```python
from build123d import *

# Parameters (mm, degrees)
BOSS_EXTRUDE1_DEPTH       = 500
SKETCH5_R                 = 1.5
CUT_EXTRUDE1_DEPTH        = 5
M5X0_8_TAPPED_HOLE1_D     = 4.2
M5X0_8_TAPPED_HOLE1_DEPTH = 10
M5X0_8_TAPPED_HOLE1_TIP   = 1.2618073


with BuildPart() as part:
    # Sketch3 → Boss-Extrude1 (new body)
    with BuildSketch(Plane(origin=(0, 0, 0), x_dir=(1, 0, 0), z_dir=(0, 1, 0))):
        with BuildLine():
            Line((-10, -16.214268408), (10, -16.214268408))
            ThreePointArc((10, -16.214268408), (0, 19.05), (-10, -16.214268408))
        make_face()
    extrude(amount=BOSS_EXTRUDE1_DEPTH)

    # Sketch5 → Cut-Extrude1 (cut)
    with BuildSketch(Plane.XY.offset(16.214268408)):
        with Locations((0, 321.4)):
            Circle(SKETCH5_R)
    extrude(amount=-CUT_EXTRUDE1_DEPTH, mode=Mode.SUBTRACT)

    # M5x0.8 Tapped Hole1
    with Locations(Plane(origin=(0, 0, 0), x_dir=(-1, 0, 0), z_dir=(0, -1, 0))):
        with Locations((0, 0)):
            Hole(M5X0_8_TAPPED_HOLE1_D / 2, depth=M5X0_8_TAPPED_HOLE1_DEPTH)
            with Locations((0, 0, -(M5X0_8_TAPPED_HOLE1_DEPTH + M5X0_8_TAPPED_HOLE1_TIP / 2))):  # 118° drill point
                Cone(0, M5X0_8_TAPPED_HOLE1_D / 2, M5X0_8_TAPPED_HOLE1_TIP, mode=Mode.SUBTRACT)


solid = part.part
```
Input: part model. Units: mm. Frame: model coordinates. Coordinates: 2 decimals unless noted, no trailing zeros. Loops run counter-clockwise (first coordinate to the right, second up) from the corner with the lowest first, then second, coordinate; pieces in that order, holes last. Notation, with made-up numbers: M -13,73.25 L 25,73.25 A18 cw 25,80.25 Z; hole C 30.25,-5 d6. An arc over 180 degrees is marked long. Use a Markdown table: item, result. Add a question column.
1) Section A-A, the plane y = 308. Return the cut outline in (x, z), plus the area to 3 significant figures.
2) Section B-B, the plane x = -15. Return the cut outline in (y, z).
3) Line query: L1, parallel to Z at x = 0, y = 3.75; L2, parallel to Y at x = 0, z = 13.4; L3, parallel to X at y = 272, z = -1.5. Output: solid intervals per line, ascending. Write a range as from..to.
4) Pin query (flat end, axial travel): P1, Ø8, axis at x = 11, y = 366, coming from the -Z side; P2, Ø1, axis at x = -3.5, y = 425, coming from the -Z side; P3, Ø1.5, axis at y = 179, z = -2.5, coming from the -X side. Return the tip coordinate at first contact, or that it passes through.
Answer below:
| question | item | result |
|---|---|---|
| 1 | outline | M -10,16.21 A19.05 ccw long 10,16.21 Z |
| 1 | area | 1,100 mm2 |
| 2 | outline | M 0,-11.74 L 500,-11.74 L 500,11.74 L 0,11.74 Z |
| 3 | L1 | -19.05..-2.1, 2.1..16.21 |
| 3 | L2 | 0..319.9, 322.9..500 |
| 3 | L3 | -18.99..18.99 |
| 4 | P1 | z = -17.72 |
| 4 | P2 | z = -18.81 |
| 4 | P3 | x = -18.97 |
